```python
from build123d import *

# Parameters (mm, degrees)
EXTRUDE_1_DEPTH     = 3
CUT_EXTRUDE_1_DEPTH = 3


with BuildPart() as part:
    # 草图1 → 凸台-拉伸1 (new body)
    with BuildSketch(Plane.XY):
        with BuildLine():
            Line((-6.425519106, 6.87161757), (2.574480894, 6.87161757))
            ThreePointArc((2.574480894, 6.87161757), (3.281587675, 6.578724351), (3.574480894, 5.87161757))
            Line((3.574480894, 5.87161757), (3.574480894, -2.12838243))
            ThreePointArc((3.574480894, -2.12838243), (3.281587675, -2.835489211), (2.574480894, -3.12838243))
            Line((2.574480894, -3.12838243), (-6.425519106, -3.12838243))
            ThreePointArc((-6.425519106, -3.12838243), (-7.132625887, -2.835489211), (-7.425519106, -2.12838243))
            Line((-7.425519106, -2.12838243), (-7.425519106, 5.87161757))
            ThreePointArc((-7.425519106, 5.87161757), (-7.132625887, 6.578724351), (-6.425519106, 6.87161757))
        make_face()
    extrude(amount=EXTRUDE_1_DEPTH)

    # 草图3 → 切除-拉伸1 (cut)
    with BuildSketch(Plane(origin=(0, 0, 0), x_dir=(-1, 0, 0), z_dir=(0, 0, -1))):
        with BuildLine():
            Line((5.425519106, -0.32838243), (5.425519106, 4.07161757))
            ThreePointArc((5.425519106, 4.07161757), (5.191204531, 4.637302995), (4.625519106, 4.87161757))
            Line((4.625519106, 4.87161757), (-0.774480894, 4.87161757))
            ThreePointArc((-0.774480894, 4.87161757), (-1.340166319, 4.637302995), (-1.574480894, 4.07161757))
            Line((-1.574480894, 4.07161757), (-1.574480894, -0.32838243))
            ThreePointArc((-1.574480894, -0.32838243), (-1.340166319, -0.894067855), (-0.774480894, -1.12838243))
            Line((-0.774480894, -1.12838243), (4.625519106, -1.12838243))
            ThreePointArc((4.625519106, -1.12838243), (5.191204531, -0.894067855), (5.425519106, -0.32838243))
        make_face()
    extrude(amount=-CUT_EXTRUDE_1_DEPTH, mode=Mode.SUBTRACT)


solid = part.part
```
Input: part model. Units: mm. Frame: model coordinates. A direction names the side the tool comes from. Coordinates: 2 decimals unless noted, no trailing zeros. Loops run counter-clockwise (first coordinate to the right, second up) from the corner with the lowest first, then second, coordinate; pieces in that order, holes last. Notation, with made-up numbers: (85, -36.5) -> (130, -36.5) arc R12 cw to (130, -23.5) -> close; hole circle Ø7 at (-20, 51.5). An arc over 180 degrees is marked (long way). Use a Markdown table: item, result.
1) Access query for faces 1 (the flat face through (-2, 6.872, 1)), 2 (the flat face through (1.574, 2, 1)). Directions: +Z, -Z, +X, -X, +Y, -Y. A direction counts if a zero-diameter tool reaches every point of the face in a straight line with its end or side. Return the directions, or none.
Results found:
| item | result |
|---|---|
| face 1 | +Z, -Z, +X, -X, +Y |
| face 2 | +Z, -Z |
2) Cut plane B-B (x = -0.5). Return the cut outline in (y, z).
Results found:
| item | result |
|---|---|
| outline | (-3.13, 0) -> (-1.13, 0) -> (-1.13, 3) -> (-3.13, 3) -> close; (4.87, 0) -> (6.87, 0) -> (6.87, 3) -> (4.87, 3) -> close |
3) Pull-direction query (Y, two-part tool) for faces 3 (the flat face through (-1.8, 5.3, 0)), 4 (the flat face through (-2, -3.128, 1)), 5 (the cylindrical face through (-5.185, -0.9, 1.479)); classes: released by +Y, released by -Y, zero draft, split by the parting line, or undercut.
Results found:
| item | result |
|---|---|
| face 3 | zero draft |
| face 4 | released by -Y |
| face 5 | undercut |
4) Contact query for a flat-ended pin moving along its axis: pin 1 (2 mm diameter, centred on x = -5.5, y = 6, fed in from -Z). Output: stop coordinate, or through.
Results found:
| item | result |
|---|---|
| pin 1 | stops at z = 0 |
5) Material intervals for line 1 along X through (y, z) = (1.25, 2.55); line 2 along Y through (x, z) = (-0.75, 1.75); line 3 along Y through (x, z) = (1, 2.75), sorted ascending. Write a range as from..to.
Results found:
| item | result |
|---|---|
| line 1 | x = -7.43..-5.43, 1.57..3.57 |
| line 2 | y = -3.13..-1.13, 4.87..6.87 |
| line 3 | y = -3.13..-1.1, 4.84..6.87 |
6) Cut plane A-A (y = 2). Return the cut outline in (x, z).
Results found:
| item | result |
|---|---|
| outline | (-7.43, 0) -> (-5.43, 0) -> (-5.43, 3) -> (-7.43, 3) -> close; (1.57, 0) -> (3.57, 0) -> (3.57, 3) -> (1.57, 3) -> close |
7) Cut plane C-C (z = 2.5). Return the cut outline in (x, y), then the cut area to 3 significant figures.
Results found:
| item | result |
|---|---|
| outline | (-7.43, -2.13) arc R1 ccw to (-6.43, -3.13) -> (2.57, -3.13) arc R1 ccw to (3.57, -2.13) -> (3.57, 5.87) arc R1 ccw to (2.57, 6.87) -> (-6.43, 6.87) arc R1 ccw to (-7.43, 5.87) -> close; hole (-5.43, -0.33) arc R0.8 ccw to (-4.63, -1.13) -> (0.77, -1.13) arc R0.8 ccw to (1.57, -0.33) -> (1.57, 4.07) arc R0.8 ccw to (0.77, 4.87) -> (-4.63, 4.87) arc R0.8 ccw to (-5.43, 4.07) -> close |
| area | 67.7 mm2 |
